Study the drawing (mm; zero at the part's minimum x, y, z) and answer. Give positions to 0.01 mm unless a question says otherwise; leave off trailing zeros. Write each loop counter-clockwise with the first axis right and the second up, starting at its lowest first coordinate (ties: lowest second). Pieces come first, ordered by that corner, then holes. Notation, with made-up numbers: M 4.25,61 L 27.25,61 A16 ccw 27.25,87 Z; hole C 53.25,23 d6. An arc over 180 degrees is marked long. Use a Markdown table: item, result. Add a question column.
Item 1: A cutting plane is placed at B-B on y = 50.5. Determine the outline of the cut face in (x, z).
Item 2: Given P1, Ø1, axis at y = 2, z = 1.5, coming from the -X side; P2, Ø1, axis at x = 75.5, z = 1.5, coming from the +Y side; P3, Ø1, axis at y = 1, z = 0.5, coming from the +X side, each flat-ended and moving along its own axis, determine where each tip first touches the part or whether it passes through.
Item 3: A cutting plane is placed at A-A on x = 53.3. Determine the outline of the cut face in (y, z).
Item 4: Consider probe 1 along Y at (x, z) = (53.3, 0.4); probe 2 along Y at (x, z) = (39, 0.4) (1 decimal); probe 3 along X at (y, z) = (69, 1.1) (1 decimal). Determine where each line is inside the solid, lowest interval first. Write a range as [from, to].
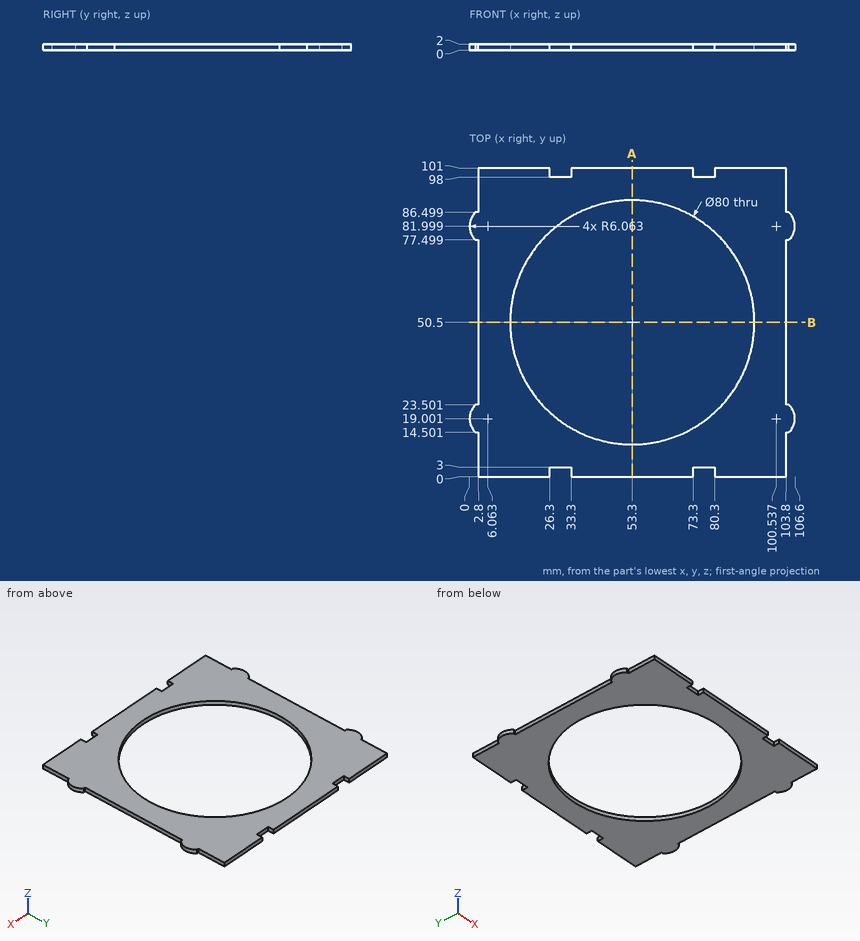
Filled in:
| question | item | result |
|---|---|---|
| 1 | outline | M 2.8,0 L 13.3,0 L 13.3,2 L 2.8,2 Z; M 93.3,0 L 103.8,0 L 103.8,2 L 93.3,2 Z |
| 2 | P1 | x = 2.8 |
| 2 | P2 | y = 98 |
| 2 | P3 | x = 103.8 |
| 3 | outline | M 0,0 L 10.5,0 L 10.5,2 L 0,2 Z; M 90.5,0 L 101,0 L 101,2 L 90.5,2 Z |
| 4 | probe 1 | [0, 10.5], [90.5, 101] |
| 4 | probe 2 | [0, 13.1], [87.9, 101] |
| 4 | probe 3 | [2.8, 17.8], [88.8, 103.8] |
